```python
from build123d import *

# Parameters (mm, degrees)
ESQUISSE1_W                  = 70
ESQUISSE1_H                  = 70
BOSS_EXTRU_1_DEPTH           = 5
BOSS_EXTRU_2_DEPTH           = 40
ENL_V_MAT_EXTRU_1_DEPTH      = 50
ESQUISSE5_R                  = 2.5
ENL_V_MAT_EXTRU_2_DEPTH      = 5
ESQUISSE6_R                  = 19
ENL_V_MAT_EXTRU_3_DEPTH      = 2
ESQUISSE7_R                  = 6.5
ENL_V_MAT_EXTRU_4_DEPTH      = 3
ESQUISSE10_R                 = 1.5
ENL_V_MAT_EXTRU_5_DEPTH      = 3
R_P_TITION_CIRCULAIRE1_COUNT = 6


with BuildPart() as part:
    # Esquisse1 → Boss.-Extru.1 (new body)
    with BuildSketch(Plane.XY):
        with Locations((-11.714867345, -1.723076923)):
            Rectangle(ESQUISSE1_W, ESQUISSE1_H)
    extrude(amount=BOSS_EXTRU_1_DEPTH)

    # Esquisse3 → Boss.-Extru.2 (add)
    with BuildSketch(Plane.XY.offset(5)):
        Polygon((-36.714867345, -36.723076923), (-36.714867345, 33.276923077), (13.285132655, 33.276923077), (13.285132655, -36.723076923), (8.285132655, -36.723076923), (8.285132655, 28.276923077), (-31.714867345, 28.276923077), (-31.714867345, -36.723076923), align=None)
    extrude(amount=BOSS_EXTRU_2_DEPTH)

    # Esquisse4 → Enlèv. mat.-Extru.1 (cut)
    with BuildSketch(Plane.ZY.offset(36.714867345)):
        Polygon((45, 28.276923077), (5, -36.723076923), (45, -36.723076923), align=None)
    extrude(amount=-ENL_V_MAT_EXTRU_1_DEPTH, mode=Mode.SUBTRACT)

    # Esquisse5 → Enlèv. mat.-Extru.2 (cut)
    with BuildSketch(Plane.XY.offset(5)):
        with Locations((-41.714867345, 13.276923077)):
            Circle(ESQUISSE5_R)
        with Locations((-41.714867345, -16.723076923)):
            Circle(ESQUISSE5_R)
        with Locations((18.285132655, -16.723076923)):
            Circle(ESQUISSE5_R)
        with Locations((18.285132655, 13.276923077)):
            Circle(ESQUISSE5_R)
    extrude(amount=-ENL_V_MAT_EXTRU_2_DEPTH, mode=Mode.SUBTRACT)

    # Esquisse6 → Enlèv. mat.-Extru.3 (cut)
    with BuildSketch(Plane.XZ.offset(-28.276923077)):
        with Locations((-11.714867345, 25)):
            Circle(ESQUISSE6_R)
    extrude(amount=-ENL_V_MAT_EXTRU_3_DEPTH, mode=Mode.SUBTRACT)

    # Esquisse7 → Enlèv. mat.-Extru.4 (cut)
    with BuildSketch(Plane.XZ.offset(-30.276923077)):
        with Locations((-11.714867345, 18)):
            Circle(ESQUISSE7_R)
    extrude(amount=-ENL_V_MAT_EXTRU_4_DEPTH, mode=Mode.SUBTRACT)

    # Esquisse10 → Enlèv. mat.-Extru.5 (cut)
    with BuildSketch(Plane.XZ.offset(-30.276923077)):
        with Locations((-26.714867345, 25)):
            Circle(ESQUISSE10_R)
    enl_v_mat_extru_5 = extrude(amount=-ENL_V_MAT_EXTRU_5_DEPTH, mode=Mode.SUBTRACT)

    # Répétition circulaire1: Enlèv. mat.-Extru.5 ×6 about axis
    r_p_tition_circulaire1_axis = Axis((-11.714867345, 0, 25), (0, 1, 0))
    for i in range(1, R_P_TITION_CIRCULAIRE1_COUNT):
        add(enl_v_mat_extru_5.rotate(r_p_tition_circulaire1_axis, i * 360 / R_P_TITION_CIRCULAIRE1_COUNT), mode=Mode.SUBTRACT)


solid = part.part
```
Work out the finished part from the listing and answer in its coordinate system (mm). A direction names the side the tool comes from. Round coordinates to 2 decimals unless told otherwise and drop trailing zeros. Write each loop counter-clockwise with the first axis right and the second up, starting at its lowest first coordinate (ties: lowest second). Pieces come first, ordered by that corner, then holes. Notation, with made-up numbers: (68, -29) - (80, -29) arc R30 cw to (80, -2) - close; hole circle Ø1 at (-4, 86). An arc over 180 degrees is marked (long way). Return JSON: item names as keys, results as strings. Group by question number.
Q1. The part is cut by section D-D on x = 11. Write down the section's boundary in (y, z).
Q2. For faces 5 (the flat face through (-36.715, 6, 20)), 6 (the flat face through (-31.715, 3, 20)), 7 (the flat face through (13.285, 7, 20)), determine the directions among +Z, -Z, +X, -X, +Y, -Y from which every point of the face is accessible in a straight line to the end or side of a thin tool.
Q3. Each of these flat-tipped pins is pushed along its axis until it touches: pin 1 Ø2.5 at (x, z) = (3.29, 25) entering from -Y; pin 2 Ø10 at (y, z) = (-8, 20) entering from +X; pin 3 Ø1 at (x, y) = (-24.5, 7.5) entering from +Z; pin 4 Ø20 at (x, z) = (-5.5, 27.5) entering from -Y. Where does it stop, or does it pass through?
Q4. Find the intervals of material crossed by L1, parallel to Y at x = 16.5, z = 3.5; L2, parallel to X at y = 7.5, z = 12; L3, parallel to Z at x = 1, y = 8.5, in increasing order.
Q5. The part is cut by section B-B on y = -15.5. Write down the section's boundary in (x, z), then the cut area to 3 significant figures.
Q6. The part is cut by section A-A on z = 18. Write down the section's boundary in (x, y).
Q7. The part is cut by section C-C on z = 38. Write down the section's boundary in (x, y).
Q8. The mould has two halves that part along Y. Classify faces 1 (the cylindrical face through (3.48, 31.756, 23.513)), 2 (the flat face through (-12, -36.723, 2)), 3 (the cylindrical face through (-44.212, -16.613, 2.535)), 4 (the cylindrical face through (-44.212, 13.387, 2.535)): released by +Y, released by -Y, zero draft, split by the parting line, or undercut.
Solved:
{
 "1": {"outline": "(-36.72, 0) - (33.28, 0) - (33.28, 45) - (28.28, 45) - (-36.72, 5) - close"},
 "2": {"face 5": "+Z, -X, +Y, -Y", "face 6": "+Z, -Y", "face 7": "+Z, +X, +Y, -Y"},
 "3": {"pin 1": "through", "pin 2": "x = 13.29", "pin 3": "z = 5", "pin 4": "y = 30.28"},
 "4": {"L1": "-36.72 to -18.47, -14.97 to 11.53, 15.03 to 33.28", "L2": "-36.71 to -31.71, 8.29 to 13.29", "L3": "0 to 5"},
 "5": {"outline": "(-46.71, 0) - (-43.9, 0) - (-43.9, 5) - (-46.71, 5) - close; (-39.53, 0) - (16.1, 0) - (16.1, 5) - (13.29, 5) - (13.29, 18.06) - (8.29, 18.06) - (8.29, 5) - (-31.71, 5) - (-31.71, 18.06) - (-36.71, 18.06) - (-36.71, 5) - (-39.53, 5) - close; (20.47, 0) - (23.29, 0) - (23.29, 5) - (20.47, 5) - close", "area": "437 mm²"},
 "6": {"outline": "(-36.71, -15.6) - (-31.71, -15.6) - (-31.71, 28.28) - (-29.38, 28.28) - (-29.38, 30.28) - (-18.21, 30.28) - (-18.21, 33.28) - (-36.71, 33.28) - close; (-5.21, 30.28) - (5.95, 30.28) - (5.95, 28.28) - (8.29, 28.28) - (8.29, -15.6) - (13.29, -15.6) - (13.29, 33.28) - (-5.21, 33.28) - close"},
 "7": {"outline": "(-36.71, 16.9) - (-31.71, 16.9) - (-31.71, 28.28) - (-25.57, 28.28) - (-25.57, 30.28) - (-20.71, 30.28) - (-20.71, 33.28) - (-36.71, 33.28) - close; (-17.71, 30.28) - (-5.71, 30.28) - (-5.71, 33.28) - (-17.71, 33.28) - close; (-2.71, 30.28) - (2.14, 30.28) - (2.14, 28.28) - (8.29, 28.28) - (8.29, 16.9) - (13.29, 16.9) - (13.29, 33.28) - (-2.71, 33.28) - close"},
 "8": {"face 1": "zero draft", "face 2": "released by -Y", "face 3": "undercut", "face 4": "undercut"}
}
